Part model, mm, in its own coordinate system. A direction names the side the tool comes from. Round coordinates to 2 decimals unless told otherwise and drop trailing zeros. Loops run counter-clockwise (first coordinate to the right, second up) from the corner with the lowest first, then second, coordinate; pieces in that order, holes last. Notation, with made-up numbers: M 5.5,26.25 L 53.5,26.25 A19 ccw 53.5,33.25 Z; hole C 11,53.25 d4. An arc over 180 degrees is marked long. Write each question's results on one line, items separated by ' | '.
from build123d import *

# Parameters (mm, degrees)
FILLET1_R          = 10
CHAMFER1_SIZE      = 5
FILLET2_R          = 15
SKETCH2_R          = 3.860242373
CUT_EXTRUDE1_DEPTH = 151


with BuildPart() as part:
    # Sketch1 → Revolve1 (revolve)
    with BuildSketch(Plane(origin=(0, 0, 0), x_dir=(1, 0, 0), z_dir=(0, 1, 0)), mode=Mode.PRIVATE) as revolve1_sk:
        Polygon((0, 0), (100, 0), (100, -50), (30, -50), (30, -150), (0, -150), align=None)
    revolve(revolve1_sk.sketch.rotate(Axis((0, 0, -26.959763618), (0, 0, 1)), 180), axis=Axis((0, 0, -26.959763618), (0, 0, 1)))  # turned: the seam where the file's is

    # Fillet1
    fillet1_edges = [part.edges().sort_by_distance(p)[0] for p in [
        (100, 0, 0),
    ]]
    fillet(fillet1_edges, radius=FILLET1_R)

    # Chamfer1
    chamfer1_edges = [part.edges().sort_by_distance(p)[0] for p in [
        (30, 0, 150),
    ]]
    chamfer(chamfer1_edges, length=CHAMFER1_SIZE)

    # Fillet2
    fillet2_edges = [part.edges().sort_by_distance(p)[0] for p in [
        (30, 0, 50),
        (100, 0, 50),
    ]]
    fillet(fillet2_edges, radius=FILLET2_R)

    # Sketch2 → Cut-Extrude1 (cut, through all)
    with BuildSketch(Plane.XY.offset(150)):
        Circle(SKETCH2_R)
    extrude(amount=-CUT_EXTRUDE1_DEPTH, mode=Mode.SUBTRACT)


solid = part.part
Item 1: Band-saw the part on D-D on z = 15.5. Give the cut face in (x, y), and give its area (3 significant figures).
Filled sheet:
outline: C 0,0 d200; hole C 0,0 d7.72 | area: 31,400 mm^2
Item 2: Two-plate mould, pull along Y, no slides. Class faces 1 (the cylindrical face through (-16.128, -25.296, 105.56)), 2 (the cylindrical face through (-0.837, -3.768, 76.05)), 3 (the flat face through (-1, 19, 0)): +Y half, -Y half, draft (parallel to the pull), parting line (faces both ways), or undercut.
Filled sheet:
face 1: parting line | face 2: undercut | face 3: draft
Item 3: Band-saw the part on A-A on x = 0. Give the cut face in (y, z), and give its area (3 significant figures).
Filled sheet:
outline: M -100,10 A10 ccw -90,0 L -3.86,0 L -3.86,150 L -25,150 L -30,145 L -30,65 A15 cw -45,50 L -85,50 A15 ccw -100,35 Z; M 3.86,0 L 90,0 A10 ccw 100,10 L 100,35 A15 ccw 85,50 L 45,50 A15 cw 30,65 L 30,145 L 25,150 L 3.86,150 Z | area: 14,800 mm^2
Item 4: Wall check: L1, parallel to Y at x = 0, z = 81; L2, parallel to Z at x = 41, y = -52.5; L3, parallel to X at y = 2.5, z = 54.5. Give the ranges that are in metal, low to high.
Filled sheet:
L1: -30 to -3.86, 3.86 to 30 | L2: 0 to 50 | L3: -34.2 to -2.94, 2.94 to 34.2
Item 5: Which spindle directions (+Z, -Z, +X, -X, +Y, -Y) get a long thin tool onto all of the face, cutting with end or side? Do faces 4 (the flat face through (-37, 37, 50)), 5 (the cylindrical face through (-95.38, -30.04, 22.68)). Say none if no direction does.
Filled sheet:
face 4: +Z | face 5: +Z, -Z
Item 6: Band-saw the part on C-C on z = 104. Give the cut face in (x, y), and give its area (3 significant figures).
Filled sheet:
outline: C 0,0 d60; hole C 0,0 d7.72 | area: 2,780 mm^2
Item 7: Drop flat-ended pins along their axis: P1, Ø4, axis at x = 54, z = 29.5, coming from the -Y side; P2, Ø6, axis at y = 3, z = 108.5, coming from the +X side; P3, Ø4, axis at x = -21.5, z = 123, coming from the +Y side. Give the stop position or say it passes through.
Filled sheet:
P1: y = -85.42 | P2: x = 30 | P3: y = 22.8
